Input: part model. Units: mm. Frame: model coordinates. A direction names the side the tool comes from. Coordinates: 2 decimals unless noted, no trailing zeros. Order: outer loops, then holes, each group sorted by start corner. A loop starts at its lowest first (then second) coordinate and runs counter-clockwise, first axis right, second up. Notation, with made-up numbers: (26, 29.25) - (75, 29.25) arc R13 cw to (75, 41.25) - close; hole circle Ø4 at (43.5, 9). An arc over 180 degrees is marked (long way). Answer as CSV lines item,"result". Start each with the question number.
Item 1: Draft query along Z for faces 1 (the cylindrical face through (-39.53, -7.9, 14.92)), 2 (the cylindrical face through (28.794, -7.902, -22.447)), 3 (the flat face through (-41.029, -8, -1)), 4 (the flat face through (38.33, -11.55, -28.59)). Return one class per face: +Z half, -Z half, draft (parallel to the pull), parting line (faces both ways), or undercut.
Item 2: Access query for faces 5 (the flat face through (31.044, -11.549, -31.765)), 6 (the flat face through (0, -3, 0)), 7 (the flat face through (37.01, -11.55, -20.01)). Directions: +Z, -Z, +X, -X, +Y, -Y. A direction counts if a zero-diameter tool reaches every point of the face in a straight line with its end or side. Return the directions, or none.
Item 3: Section B-B (z = 10.35). Output: boundary loops of the cut face in (x, y).
Item 4: Material intervals for line 1 along X through (y, z) = (-9, -15); line 2 along X through (y, z) = (-2.5, -21); line 3 along Z through (x, y) = (-15, -5.25), sorted ascending.
Item 5: Section A-A (x = -34.5). Output: boundary loops of the cut face in (y, z).
Item 6: Section C-C (y = -11.75). Output: boundary loops of the cut face in (x, z), and give its area (3 significant figures).
Item 7: Section D-D (x = -20.5). Output: boundary loops of the cut face in (y, z).
Item 8: First-contact query: pin 1 (5 mm diameter, centred on y = -12, z = -20.5, fed in from -X); pin 2 (5 mm diameter, centred on x = 25.5, y = -4, fed in from -Z); pin 3 (1 mm diameter, centred on y = -8.5, z = -34.5, fed in from -X); pin 4 (5 mm diameter, centred on x = 5, z = 0, fed in from +Y). Flat tips, straight axial feed; report the tip coordinate or a pass-through.
from build123d import *

# Parameters (mm, degrees)
EXTRUDE_1_DEPTH        = 14
EXTRUDE_2_DEPTH        = 7
CUT_EXTRUDE_1_DEPTH    = 41.028932
CUT_EXTRUDE_2_DEPTH    = 38.1
HOLE_WIZARD_M4_1_D     = 4.318
HOLE_WIZARD_M4_1_DEPTH = 14
FILLET_1_R             = 5
FILLET_3_R             = 1.27
FILLET_4_R             = 1.27


with BuildPart() as part:
    # 草图1 → 凸台-拉伸1 (new body)
    with BuildSketch(Plane.XZ.offset(15)):
        Polygon((4.743453, -52.27499), (35.219756, -21.798688), (-2.928932, 16.35), (-41.028932, 16.35), (-41.028932, -16.35), align=None)
    extrude(amount=-EXTRUDE_1_DEPTH)

    # 草图2 → 凸台-拉伸2 (add)
    with BuildSketch(Plane.XZ.offset(15)):
        Polygon((43.705037, -23.212901), (38.75529, -18.263154), (35.219756, -21.798688), (28.148688, -28.869756), (33.098435, -33.819503), align=None)
    extrude(amount=-EXTRUDE_2_DEPTH)

    # 草图3 → 切除-拉伸1 (cut)
    with BuildSketch(Plane.ZY.offset(41.028932)):
        with BuildLine():
            Line((6.270766, -1), (-6.270766, -1))
            ThreePointArc((-6.270766, -1), (0, -6.35), (6.270766, -1))
        make_face()
    extrude(amount=-CUT_EXTRUDE_1_DEPTH, mode=Mode.SUBTRACT)

    # 草图4 → 切除-拉伸2 (cut)
    with BuildSketch(Plane(origin=(6.710534, 0, 6.710534), x_dir=(0.707107, 0, -0.707107), z_dir=(0.707107, 0, 0.707107))):
        with BuildLine():
            Line((30.270005, -1), (9.538252, -1))
            ThreePointArc((9.538252, -1), (19.904128, -10.414), (30.270005, -1))
        make_face()
    extrude(amount=-CUT_EXTRUDE_2_DEPTH, mode=Mode.SUBTRACT)

    # M4 间隙孔1
    with Locations(Plane(origin=(0, -15, 0), x_dir=(-1, 0, 0), z_dir=(0, -1, 0))):
        with Locations((35.028932, -10.35), (-5, 0), (15, 15), (12.103043, -10.35), (35.028932, 10.35), (-4.743453, 43.789709), (-26.734474, 21.798688)):
            Hole(HOLE_WIZARD_M4_1_D / 2, depth=HOLE_WIZARD_M4_1_DEPTH)

    # 圆角1
    fillet_1_edges = [part.edges().sort_by_distance(p)[0] for p in [
        (-41.028932, -8, -16.35),
        (-41.028932, -8, 16.35),
        (-2.928932, -8, 16.35),
        (4.743453, -8, -52.27499),
    ]]
    fillet(fillet_1_edges, radius=FILLET_1_R)

    # 圆角3
    fillet_3_edges = [part.edges().sort_by_distance(p)[0] for p in [
        (31.684222, -8, -25.334222),
    ]]
    fillet(fillet_3_edges, radius=FILLET_3_R)

    # 圆角4
    fillet_4_edges = [part.edges().sort_by_distance(p)[0] for p in [
        (28.148688, -11.5, -28.869756),
    ]]
    fillet(fillet_4_edges, radius=FILLET_4_R)


solid = part.part
Determined:
1,face 1,"+Z half"
1,face 2,"undercut"
1,face 3,"draft"
1,face 4,"-Z half"
2,face 5,"-Z, +Y, -Y"
2,face 6,"-X, +Y"
2,face 7,"+Z, +Y, -Y"
3,outline,"(-41.03, -15) - (-37.19, -15) - (-37.19, -1) - (-41.03, -1) - close; (-32.87, -15) - (-14.26, -15) - (-14.26, -1) - (-32.87, -1) - close; (-9.94, -15) - (3.07, -15) - (3.07, -1) - (-9.94, -1) - close"
4,line 1,"x = -40.91 to -17.16, -12.84 to 5.74, 20.56 to 28.42"
4,line 2,"x = -35.1 to -7.15, 21.45 to 24.73, 28.74 to 34.42"
4,line 3,"z = -36.78 to -17.16, -12.84 to -3.57, 3.57 to 16.35"
5,outline,"(-15, -21.47) - (-1, -21.47) - (-1, -12.44) - (-15, -12.44) - close; (-15, -8.26) - (-1, -8.26) - (-1, -6.27) arc R6.35 cw to (-1, 6.27) - (-1, 8.26) - (-15, 8.26) - close; (-15, 12.44) - (-1, 12.44) - (-1, 16.35) - (-15, 16.35) - close"
6,outline,"(-41.03, -13.92) arc R5 ccw to (-39.12, -17.85) - (1.26, -49.54) arc R5 ccw to (7.88, -49.14) - (27.25, -29.77) arc R1.27 cw to (29.05, -29.77) - (33.1, -33.82) - (43.71, -23.21) - (38.76, -18.26) - (35.22, -21.8) - (-1.46, 14.89) arc R5 ccw to (-5, 16.35) - (-36.03, 16.35) arc R5 ccw to (-41.03, 11.35) - close; hole circle Ø4.32 at (-35.03, -10.35); hole circle Ø4.32 at (-35.03, 10.35); hole circle Ø4.32 at (-15, -15); hole circle Ø4.32 at (-12.1, 10.35); hole circle Ø4.32 at (4.74, -43.79); hole circle Ø4.32 at (5, 0); hole circle Ø4.32 at (26.73, -21.8)"
6,area,"3,210 mm^2"
7,outline,"(-15, -32.46) - (-1, -32.46) - (-1, -6.27) arc R6.35 cw to (-1, 6.27) - (-1, 16.35) - (-15, 16.35) - close"
8,pin 1,"stops at x = -38.93"
8,pin 2,"stops at z = -34.02"
8,pin 3,"stops at x = -18.54"
8,pin 4,"stops at y = -1"
